Design review of the part built by this model. Coordinates are the model's own, in mm. A direction names the side the tool comes from. Give positions to 0.01 mm unless a question says otherwise; leave off trailing zeros. Loops run counter-clockwise (first coordinate to the right, second up) from the corner with the lowest first, then second, coordinate; pieces in that order, holes last. Notation, with made-up numbers: (78.25, 48.25) -> (86.25, 48.25) arc R10 cw to (86.25, 66.25) -> close; hole circle Ø11 at (47.25, 45). An arc over 180 degrees is marked (long way). Answer as CSV lines item,"result".
from build123d import *

# Parameters (mm, degrees)
EXTRUSION1_DEPTH        = 64
COQUE14_T               = 8
EXTRUSION2_DEPTH        = 71
ENL_V_MAT_EXTRU_1_DEPTH = 65
ESQUISSE8_R             = 26.5
EXTRUSION3_DEPTH        = 84
ESQUISSE9_R             = 34.5
EXTRUSION4_DEPTH        = 14
ESQUISSE10_R            = 26.5
EXTRUSION5_DEPTH        = 82
ESQUISSE11_R            = 30
EXTRUSION6_DEPTH        = 70
ESQUISSE12_R            = 25
EXTRUSION7_DEPTH        = 110
ESQUISSE13_R            = 17.5
EXTRUSION8_DEPTH        = 50
ESQUISSE14_R            = 10
ENL_V_MAT_EXTRU_2_DEPTH = 523.264300905


with BuildPart() as part:
    # Esquisse1 → Extrusion1 (new body)
    with BuildSketch(Plane.XY):
        with BuildLine():
            Line((53, -141), (85, -141))
            Line((85, -141), (85, 0))
            ThreePointArc((85, 0), (0, 85), (-85, 0))
            Line((-85, 0), (-85, -141))
            Line((-85, -141), (-53, -141))
            ThreePointArc((-53, -141), (0, -194), (53, -141))
        make_face()
    extrude(amount=EXTRUSION1_DEPTH)

    # Coque14
    coque14_openings = [part.faces().sort_by_distance(p)[0] for p in [
        (0, -50.38495727, 0),
    ]]
    offset(amount=COQUE14_T, openings=coque14_openings, kind=Kind.INTERSECTION)

    # Esquisse2 → Extrusion2 (add)
    with BuildSketch(Plane(origin=(0, -139, 0), x_dir=(-1, 0, 0), z_dir=(0, 1, 0))):
        with BuildLine():
            Line((-81, 72), (-81, 353))
            ThreePointArc((-81, 353), (-30.212730552, 428.154447058), (58.461504015, 409.0647175))
            Line((58.461504015, 409.0647175), (134.365601194, 329.915693302))
            ThreePointArc((134.365601194, 329.915693302), (146.818305394, 306.69624557), (145.44507462, 280.384141281))
            Line((145.44507462, 280.384141281), (75.381729126, 72))
            Line((75.381729126, 72), (-81, 72))
        make_face()
    extrude(amount=EXTRUSION2_DEPTH)

    # Esquisse4 → Enlèv. mat.-Extru.1 (cut)
    with BuildSketch(Plane(origin=(-53, -141, 64), x_dir=(1, 0, 0), z_dir=(0, -1, 0))):
        Polygon((101.5, 8), (101.5, 173), (53, 188), (4.5, 173), (4.5, 8), align=None)
    extrude(amount=-ENL_V_MAT_EXTRU_1_DEPTH, mode=Mode.SUBTRACT)

    # Esquisse8 → Extrusion3 (add)
    with BuildSketch(Plane.XZ.offset(139)):
        with Locations(Location((-99, 296, 0), (0, 0, 90))):
            Circle(ESQUISSE8_R)
    extrude(amount=EXTRUSION3_DEPTH)

    # Esquisse9 → Extrusion4 (add)
    with BuildSketch(Plane.XZ.offset(223)):
        with Locations(Location((-99, 296, 0), (0, 0, 270))):
            Circle(ESQUISSE9_R)
    extrude(amount=EXTRUSION4_DEPTH)

    # Esquisse10 → Extrusion5 (add)
    with BuildSketch(Plane.XZ.offset(237)):
        with Locations(Location((-99, 296, 0), (0, 0, 90))):
            Circle(ESQUISSE10_R)
    extrude(amount=EXTRUSION5_DEPTH)

    # Esquisse11 → Extrusion6 (add)
    with BuildSketch(Plane.XZ.offset(319)):
        with Locations(Location((-99, 296, 0), (0, 0, 270))):
            Circle(ESQUISSE11_R)
    extrude(amount=EXTRUSION6_DEPTH)

    # Esquisse12 → Extrusion7 (add)
    with BuildSketch(Plane.XY.offset(72)):
        with Locations((0, -141)):
            Circle(ESQUISSE12_R)
    extrude(amount=EXTRUSION7_DEPTH)

    # Esquisse13 → Extrusion8 (add)
    with BuildSketch(Plane.XY.offset(182)):
        with Locations((0, -141)):
            Circle(ESQUISSE13_R)
    extrude(amount=EXTRUSION8_DEPTH)

    # Esquisse14 → Enlèv. mat.-Extru.2 (cut, through all)
    with BuildSketch(Plane.XZ.offset(139)):
        with Locations(Location((0, 353, 0), (0, 0, 270))):
            Circle(ESQUISSE14_R)
    extrude(amount=-ENL_V_MAT_EXTRU_2_DEPTH, mode=Mode.SUBTRACT)


solid = part.part
Q1. Clearance check with flat-ended pins moving along their axes: pin 1 Ø10 at (y, z) = (-143, 326) entering from -X; pin 2 Ø10 at (x, y) = (-97, -236.5) entering from +Z; pin 3 Ø3 at (x, y) = (-109.5, -119.5) entering from +Z. State where each tip first meets the part, or that it passes through.
Filled sheet:
pin 1,"stops at x = -139.89"
pin 2,"stops at z = 330.5"
pin 3,"stops at z = 357.41"
Q2. We need section C-C, the plane z = 164.5. State the section outline as (x, y) points, and give its area (3 significant figures).
Filled sheet:
outline,"(-106.48, -139) -> (-48.5, -139) -> (-48.5, -76) -> (48.5, -76) -> (48.5, -139) -> (81, -139) -> (81, -68) -> (-106.48, -68) -> close; circle Ø50 at (0, -141)"
area,"9,160 mm^2"
Q3. For faces 4 (the flat face through (81, -104, 211)), 5 (the flat face through (-1, -52, 72)), 6 (the flat face through (0, -141, 232)), list the 3-axis set-ups (+Z, -Z, +X, -X, +Y, -Y) from which the entire face can be reached by the end or side of a thin tool; tool diameter is ignored.
Filled sheet:
face 4,"+Z, +X, +Y, -Y"
face 5,"none"
face 6,"-Y"
Q4. We need section D-D, the plane x = 34.5. State the section outline as (y, z) points.
Filled sheet:
outline,"(-191.31, 0) -> (-181.23, 0) -> (-181.23, 64) -> (77.68, 64) -> (77.68, 0) -> (86.36, 0) -> (86.36, 72) -> (-68, 72) -> (-68, 426.29) -> (-139, 426.29) -> (-139, 241.33) -> (-76, 241.33) -> (-76, 72) -> (-191.31, 72) -> close"
Q5. To check wall thickness, follow probe 1 along Y at (x, z) = (65.5, 290); probe 2 along X at (y, z) = (-105, 353); probe 3 along X at (y, z) = (-166.5, 32.5). State the ranges of each line that lie inside material, in increasing order. Write a range as from..to.
Filled sheet:
probe 1,"y = -139..-68"
probe 2,"x = -112.23..-10, 10..81"
probe 3,"x = -55.41..-46.46, 46.46..55.41"
Q6. The part is to be moulded in two halves that separate along X. For faces 1 (the cylindrical face through (1.87, 84.98, 31.55)), 2 (the cylindrical face through (-146.735, -103.997, 307.06)), 3 (the cylindrical face through (-100.165, -277.426, 269.526)), say which applies: pulls with the +X half, pulls with the -X half, needs draft (parallel to the pull), parting line crosses it, or undercut.
Filled sheet:
face 1,"undercut"
face 2,"pulls with the -X half"
face 3,"parting line crosses it"
Q7. We need section A-A, the plane y = -28. State the section outline as (x, z) points.
Filled sheet:
outline,"(-93, 0) -> (-85, 0) -> (-85, 64) -> (85, 64) -> (85, 0) -> (93, 0) -> (93, 72) -> (-93, 72) -> close"
Q8. We need section B-B, the plane y = -108. State the section outline as (x, z) points.
Filled sheet:
outline,"(-145.45, 280.38) -> (-75.38, 72) -> (-93, 72) -> (-93, 0) -> (-85, 0) -> (-85, 64) -> (85, 64) -> (85, 0) -> (93, 0) -> (93, 72) -> (81, 72) -> (81, 353) arc R81 ccw to (-58.46, 409.06) -> (-134.37, 329.92) arc R49 ccw to start; hole (-48.5, 72) -> (48.5, 72) -> (48.5, 237) -> (0, 252) -> (-48.5, 237) -> close; hole circle Ø20 at (0, 353)"
